Verification items for the finished model (mm, model axes). Face numbers are marked on the shaded views. A direction names the side the tool comes from. Coordinates: 2 decimals unless noted, no trailing zeros. Order: outer loops, then holes, each group sorted by start corner. A loop starts at its lowest first (then second) coordinate and runs counter-clockwise, first axis right, second up. Notation, with made-up numbers: (-19, 23.25) -> (13, 23.25) arc R6 cw to (13, 31.25) -> close; hole circle Ø1 at (34.5, 3). An arc over 180 degrees is marked (long way). Write item = value, one per line. Start each with the question number.
1. Cross-section at D-D on x = 52. Record the cut outline in (y, z).
2. Thickness scan on line 1 along X through (y, z) = (23, -54); line 2 along Z through (x, y) = (32.5, 7); line 3 along Z through (x, y) = (62.5, 13). Record the ranges inside material, lowest first. Write a range as from..to.
3. Go/stop test with flat-tipped pins: P1, Ø11.5, axis at x = 16, y = 20.5, coming from the -Z side; P2, Ø7.5, axis at y = 9.52, z = -49.2, coming from the -X side; P3, Ø6, axis at y = 5, z = -14.5, coming from the -X side. Record where each tip stops, or that it passes through.
4. Set-up check for the marked faces 1 and 2: record each of +Z, -Z, +X, -X, +Y, -Y from which the full face is reachable in a straight line by a thin tool's end or side.
5. Cross-section at C-C on z = -49. Record the cut outline in (x, y), plus the area to 3 significant figures.
6. Cross-section at B-B on y = 11. Record the cut outline in (x, z).
7. Cross-section at A-A on x = 15.24. Record the cut outline in (y, z).
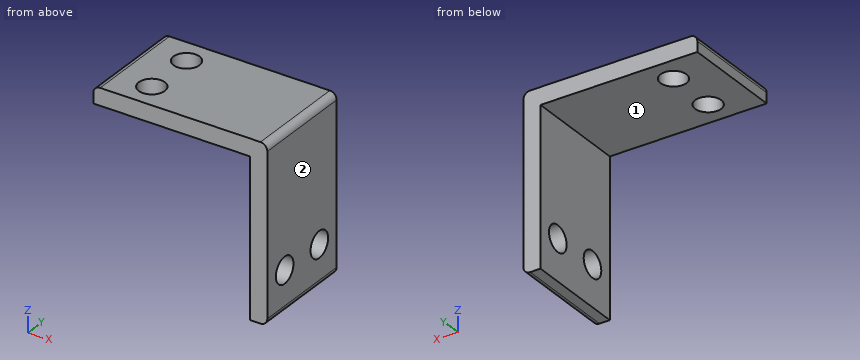
from build123d import *

# Parameters (mm, degrees)
SKETCH1_W           = 64.4398
SKETCH1_H           = 38.1
BOSS_EXTRUDE1_DEPTH = 6.35
SKETCH2_W           = 64.4398
SKETCH2_H           = 38.1
BOSS_EXTRUDE2_DEPTH = 6.35
SKETCH3_R           = 4.826
CUT_EXTRUDE1_DEPTH  = 99.775430387
SKETCH4_R           = 4.826
CUT_EXTRUDE4_DEPTH  = 99.775430387
FILLET1_R           = 2.54
FILLET2_R           = 2.54
FILLET3_R           = 2.54


with BuildPart() as part:
    # Sketch1 → Boss-Extrude1 (new body)
    with BuildSketch(Plane.XY):
        with Locations((32.2199, 19.05)):
            Rectangle(SKETCH1_W, SKETCH1_H)
    extrude(amount=-BOSS_EXTRUDE1_DEPTH)

    # Sketch2 → Boss-Extrude2 (add)
    with BuildSketch(Plane(origin=(64.4398, 0, 0), x_dir=(0, 0, -1), z_dir=(1, 0, 0))):
        with Locations((32.2199, 19.05)):
            Rectangle(SKETCH2_W, SKETCH2_H)
    extrude(amount=-BOSS_EXTRUDE2_DEPTH)

    # Sketch3 → Cut-Extrude1 (cut, through all)
    with BuildSketch(Plane(origin=(64.4398, 0, 0), x_dir=(0, 0, -1), z_dir=(1, 0, 0))):
        with Locations((49.1998, 28.575)):
            Circle(SKETCH3_R)
        with Locations(Location((49.1998, 9.525, 0), (0, 0, 180))):
            Circle(SKETCH3_R)
    extrude(amount=-CUT_EXTRUDE1_DEPTH, mode=Mode.SUBTRACT)

    # Sketch4 → Cut-Extrude4 (cut, through all)
    with BuildSketch(Plane.XY):
        with Locations((15.24, 28.575)):
            Circle(SKETCH4_R)
        with Locations(Location((15.24, 9.525, 0), (0, 0, 180))):
            Circle(SKETCH4_R)
    extrude(amount=-CUT_EXTRUDE4_DEPTH, mode=Mode.SUBTRACT)

    # Fillet1
    fillet1_edges = [part.edges().sort_by_distance(p)[0] for p in [
        (0, 19.05, 0),
    ]]
    fillet(fillet1_edges, radius=FILLET1_R)

    # Fillet2
    fillet2_edges = [part.edges().sort_by_distance(p)[0] for p in [
        (64.4398, 19.05, -64.4398),
    ]]
    fillet(fillet2_edges, radius=FILLET2_R)

    # Fillet3
    fillet3_edges = [part.edges().sort_by_distance(p)[0] for p in [
        (64.4398, 19.05, 0),
    ]]
    fillet(fillet3_edges, radius=FILLET3_R)


solid = part.part
Worked out:
q1.outline = (0, -6.35) -> (38.1, -6.35) -> (38.1, 0) -> (0, 0) -> close
q2.line_1 = 58.09..64.44
q2.line_2 = -6.35..0
q2.line_3 = -64.37..-52.55, -45.85..-0.07
q3.P1 = -6.35
q3.P2 = through
q3.P3 = 58.09
q4.face_1 = -Z, -X, +Y, -Y
q4.face_2 = +Z, -Z, +X, +Y, -Y
q5.outline = (58.09, 0) -> (64.44, 0) -> (64.44, 4.7) -> (58.09, 4.7) -> close; (58.09, 14.35) -> (64.44, 14.35) -> (64.44, 23.75) -> (58.09, 23.75) -> close; (58.09, 33.4) -> (64.44, 33.4) -> (64.44, 38.1) -> (58.09, 38.1) -> close
q5.area = 119 mm²
q6.outline = (0, -6.35) -> (10.64, -6.35) -> (10.64, 0) -> (2.54, 0) arc R2.54 ccw to (0, -2.54) -> close; (19.84, -6.35) -> (58.09, -6.35) -> (58.09, -44.6) -> (64.44, -44.6) -> (64.44, -2.54) arc R2.54 ccw to (61.9, 0) -> (19.84, 0) -> close; (58.09, -64.44) -> (61.9, -64.44) arc R2.54 ccw to (64.44, -61.9) -> (64.44, -53.79) -> (58.09, -53.79) -> close
q7.outline = (0, -6.35) -> (4.7, -6.35) -> (4.7, 0) -> (0, 0) -> close; (14.35, -6.35) -> (23.75, -6.35) -> (23.75, 0) -> (14.35, 0) -> close; (33.4, -6.35) -> (38.1, -6.35) -> (38.1, 0) -> (33.4, 0) -> close
